```python
from build123d import *

# Parameters (mm, degrees)
ESQUISSE1_W                  = 52
ESQUISSE1_H                  = 3
CHANFREIN1_SIZE              = 0.5
ENL_V_MAT_EXTRU_1_DEPTH      = 27.343879745
ENL_V_MAT_EXTRU_1_DEPTH_BACK = 27.343879745
ESQUISSE2_W                  = 4
ESQUISSE2_H                  = 2
ESQUISSE3_W                  = 0.74
ESQUISSE3_H                  = 1


with BuildPart() as part:
    # Esquisse1 → Révolution1 (revolve)
    with BuildSketch(Plane.XY, mode=Mode.PRIVATE) as r_volution1_sk:
        with Locations((0, 1.5)):
            Rectangle(ESQUISSE1_W, ESQUISSE1_H)
    revolve(r_volution1_sk.sketch.rotate(Axis((0, 0, 0), (1, 0, 0)), 90), axis=Axis((0, 0, 0), (1, 0, 0)))

    # Chanfrein1
    chanfrein1_edges = [part.edges().sort_by_distance(p)[0] for p in [
        (26, 0, -3),
        (-26, 0, -3),
    ]]
    chamfer(chanfrein1_edges, length=CHANFREIN1_SIZE)

    # Esquisse2 → Enlèv. mat.-Extru.1 (cut, two sides: drawn at the far end of the back side and taken through both)
    with BuildSketch(Plane.XY.offset(-ENL_V_MAT_EXTRU_1_DEPTH_BACK)):
        with Locations((-8.1, 3)):
            Rectangle(ESQUISSE2_W, ESQUISSE2_H)
    extrude(amount=ENL_V_MAT_EXTRU_1_DEPTH + ENL_V_MAT_EXTRU_1_DEPTH_BACK, mode=Mode.SUBTRACT)

    # Esquisse3 → Enlèvement de matière-Révolution1 (revolve, cut)
    with BuildSketch(Plane.XY):
        with Locations((-21.03, 2.5)):
            Rectangle(ESQUISSE3_W, ESQUISSE3_H)
        with Locations((21.03, 2.5)):
            Rectangle(ESQUISSE3_W, ESQUISSE3_H)
    revolve(axis=Axis((0, 0, 0), (-1, 0, 0)), mode=Mode.SUBTRACT)


solid = part.part
```
Work out the finished part from the listing and answer in its coordinate system (mm). A direction names the side the tool comes from. Give positions to 0.01 mm unless a question says otherwise; leave off trailing zeros. Order: outer loops, then holes, each group sorted by start corner. A loop starts at its lowest first (then second) coordinate and runs counter-clockwise, first axis right, second up. Notation, with made-up numbers: (28, 28.25) - (86, 28.25) arc R21 ccw to (86, 61.25) - close; hole circle Ø6 at (-33.75, 64). An arc over 180 degrees is marked (long way). One line per item, written item: value. Start each with the question number.
1. Consider line 1 (X direction, y = -1.5, z = 1.75); line 2 (X direction, y = 2.5, z = 0); line 3 (X direction, y = -2, z = -2). Determine where each line is inside the solid, lowest interval first.
2. Which of the six approach directions +Z, -Z, +X, -X, +Y, -Y give full straight-line access (tool end or side, diameter ignored) to faces 4 (the face through (-10.1, 2.4, 0)), 5 (the face through (21.4, -2, 1)), 6 (the face through (23.48, 1.15, 2.77))?
3. For a pull along X with two mould halves and no side action, classify faces 1 (the face through (0, -3, 0)), 2 (the face through (-8, 2, 0)), 3 (the face through (26, 0, 0)) as released by +X, released by -X, zero draft, split by the parting line, or undercut.
4. Section B-B, the plane x = -8 is taken. Write down the section's boundary in (y, z).
5. Each of these flat-tipped pins is pushed along its axis until it touches: pin 1 Ø3 at (x, z) = (-7.5, 0.5) entering from +Y; pin 2 Ø2 at (x, y) = (20, -1.5) entering from -Z; pin 3 Ø1 at (x, y) = (10, 1) entering from +Z. Where does it stop, or does it pass through?
6. Section A-A, the plane z = 0 is taken. Write down the section's boundary in (x, y).
Filled sheet:
1. line 1: -26 to -21.4, -20.66 to 20.66, 21.4 to 26
1. line 2: -26 to -21.4, -20.66 to -10.1, -6.1 to 20.66, 21.4 to 26
1. line 3: -25.67 to -21.4, -20.66 to 20.66, 21.4 to 25.67
2. face 4: +Z, -Z, +Y
2. face 5: none
2. face 6: +X, -X
3. face 1: zero draft
3. face 2: undercut
3. face 3: released by +X
4. outline: (2, -2.24) - (2, 2.24) arc R3 ccw (long way) to start
5. pin 1: y = 3
5. pin 2: z = -2.96
5. pin 3: z = 2.96
6. outline: (-26, -2.5) - (-25.5, -3) - (-21.4, -3) - (-21.4, -2) - (-20.66, -2) - (-20.66, -3) - (20.66, -3) - (20.66, -2) - (21.4, -2) - (21.4, -3) - (25.5, -3) - (26, -2.5) - (26, 2.5) - (25.5, 3) - (21.4, 3) - (21.4, 2) - (20.66, 2) - (20.66, 3) - (-6.1, 3) - (-6.1, 2) - (-10.1, 2) - (-10.1, 3) - (-20.66, 3) - (-20.66, 2) - (-21.4, 2) - (-21.4, 3) - (-25.5, 3) - (-26, 2.5) - close
